Here's how the part is built. I have some questions about the finished solid (model axes, mm). A direction names the side the tool comes from. Coordinates: 2 decimals unless noted, no trailing zeros. Loops run counter-clockwise (first coordinate to the right, second up) from the corner with the lowest first, then second, coordinate; pieces in that order, holes last. Notation, with made-up numbers: (-13, 34.25) -> (25, 34.25) arc R20 ccw to (25, 56.25) -> close; hole circle Ø6 at (38, -37.75). An arc over 180 degrees is marked (long way). Answer as a JSON object with one key per item and string values. Group by question number.
Q1. On a 3-axis mill with a long thin cutter (end or side, diameter ignored), from which of +Z, -Z, +X, -X, +Y, -Y can I reach the whole of each face in a straight line? I mean faces 1 (the flat face through (1.75, 0, -1)), 2 (the flat face through (-1.75, 0, -1)), 3 (the flat face through (0, 0, -25.1)), 4 (the cylindrical face through (2, 0, -9)). Say none if no direction works.
Q2. I want a section at A-A on z = -4.5. Write out the boundary of the cut face in (x, y).
Q3. I need wall thicknesses on line 1 (Y direction, x = -0.05, z = -4.5); line 2 (X direction, y = 0.1, z = -22.5). Which ranges of each line are inside material? Lowest first, please.
Q4. I want a section at B-B on z = -19. Write out the boundary of the cut face in (x, y), then the cut area to 3 significant figures.
Q5. I'm going to push flat-ended pins straight in: pin 1 (1 mm diameter, centred on y = -0.5, z = -1.5, fed in from -X); pin 2 (0.6 mm diameter, centred on y = -0.5, z = -1.5, fed in from +X). Where does each tip first touch, or does it pass through?
Q6. I want a section at C-C on z = -7.75. Write out the boundary of the cut face in (x, y), then the cut area to 3 significant figures.
Q7. Thinking about a two-plate mould opening in Y: for faces 5 (the cylindrical face through (0, -3, -21)), 6 (the conical face through (-0.05, 0.17, -6.48)), 7 (the flat face through (-2, 1, -17)), which applies, released by +Y, released by -Y, zero draft, split by the parting line, or undercut?
Autodesk Inventor part; units mm, degrees
ref_plane "ANBAU_XY" through (0, 0, -25.1) normal (0, 0, -1) x (1, 0, 0)
ref_plane "ANBAU_YZ" through (0, 0, -25.1) normal (1, 0, 0) x (0, -1, 0)
ref_plane "ANBAU_ZX" through (0, 0, -25.1) normal (0, -1, 0) x (0, 0, -1)
sketch "Sketch_1" plane through (0, 0, 0) normal (1, 0, 0) x (0, 1, 0)
  line L0 (0, -25.1) -> (0, -6.5811)
  line L1 (0, -6.5811) -> (1.0065, -6)
  line L2 (1.0065, -6) -> (1.0065, -0.2435)
  line L3 (1.0065, -0.2435) -> (1.25, 0)
  line L4 (1.25, 0) -> (1.8, 0)
  line L5 (1.8, 0) -> (2, -0.2)
  line L6 (2, -0.2) -> (2, -17)
  line L7 (2, -17) -> (3, -17)
  line L8 (3, -17) -> (3, -25.1)
  line L9 (3, -25.1) -> (0, -25.1)
  line L10 (0, -25.1) -> (0, -6.5811)
revolve "Revolution1" add sketch "Sketch_1" angle 360 about axis through (0, 0, -25.1) along (0, 0, -1)
thread "Thread1"
sketch "Sketch_2" plane through (0, 0, 0) normal (0, 0, 1) x (1, 0, 0)
  line L0 (-3.5, 15) -> (-3.5, -15)
  line L1 (-3.5, -15) -> (3.5, -15)
  line L2 (3.5, -15) -> (3.5, 15)
  line L3 (3.5, 15) -> (-3.5, 15)
  line L4 (-1.75, 10) -> (-1.75, -10)
  line L5 (-1.75, -10) -> (1.75, -10)
  line L6 (1.75, -10) -> (1.75, 10)
  line L7 (1.75, 10) -> (-1.75, 10)
extrude "Extrusion1" cut sketch "Sketch_2" against normal blind 2.7
ref_plane "ANBAU_XY" through (0, 0, -25.1) normal (0, 0, -1) x (1, 0, 0)
ref_plane "ANBAU_YZ" through (0, 0, -25.1) normal (1, 0, 0) x (0, -1, 0)
ref_plane "ANBAU_ZX" through (0, 0, -25.1) normal (0, -1, 0) x (0, 0, -1)
properties part number "5267300 AEN-S-6-5-I-A---(highP)"
Result set:
{
 "1": {"face 1": "+Z, +X, +Y, -Y", "face 2": "+Z, -X, +Y, -Y", "face 3": "-Z, +X, -X, +Y, -Y", "face 4": "+Z"},
 "2": {"outline": "circle Ø4 at (0, 0); hole circle Ø2.01 at (0, 0)"},
 "3": {"line 1": "y = -2 to -1.01, 1.01 to 2", "line 2": "x = -3 to 3"},
 "4": {"outline": "circle Ø6 at (0, 0)", "area": "28.3 mm²"},
 "5": {"pin 1": "stops at x = -1.75", "pin 2": "stops at x = 1.75"},
 "6": {"outline": "circle Ø4 at (0, 0)", "area": "12.6 mm²"},
 "7": {"face 5": "split by the parting line", "face 6": "undercut", "face 7": "zero draft"}
}
